Read the model definition and answer for the solid it produces. Units are mm, in the model's axes. A direction names the side the tool comes from. Coordinates: 2 decimals unless noted, no trailing zeros. Write each loop counter-clockwise with the first axis right and the second up, starting at its lowest first coordinate (ties: lowest second). Pieces come first, ordered by that corner, then holes.
(1) Section B-B on z = 63.5 is taken. Write down the section's boundary in (x, y).
(2) Find the intervals of material crossed by probe 1 along Y at (x, z) = (44.5, 27); probe 2 along X at (y, z) = (6, -31); probe 3 along Z at (x, y) = (39, 6), in increasing order.
(3) Which of the six approach directions +Z, -Z, +X, -X, +Y, -Y give full straight-line access (tool end or side, diameter ignored) to faces 1 (the flat face through (25.222, 99.563, -12.21)), 2 (the flat face through (25.49, 77.21, -13.04)), 3 (the flat face through (12.7, 102, -8)), 4 (the flat face through (38.1, 77, -12)), 5 (the flat face through (27.686, 159, 17))?
(4) Given pin 1 (1.6 mm diameter, centred on x = 19, y = 186, fed in from +Z); pin 2 (2 mm diameter, centred on y = 101, z = -7, fed in from +X); pin 3 (5 mm diameter, centred on x = 43.5, z = -43.5, fed in from +Y); pin 4 (1 mm diameter, centred on x = -2, z = -3, fed in from -Y), each flat-ended and moving along its own axis, determine where each tip first touches the part or whether it passes through.
(5) The mould has two halves that part along X. Classify faces 6 (the flat face through (25.22, 74.51, -16.39)), 7 (the cylindrical face through (14.149, 78.337, -20.316)), 8 (the flat face through (19.05, 77, -10)), 9 (the flat face through (31.75, 102, -6)): +X half, -X half, draft (parallel to the pull), parting line (faces both ways), or undercut.
(6) Section A-A on x = 4 is taken. Write down the section's boundary in (y, z) (1 decimal), then the cut area to 3 significant figures.
from build123d import *

# Parameters (mm, degrees)
F1_DEPTH  = 50.8
F2_R      = 31.75
F3_DEPTH  = 50.8
F4_R      = 17.78
F5_R      = 7.62
F6_R      = 1.5875
F7_DEPTH  = 4.7625
F8_W      = 4.572
F8_H      = 86.36
F9_DEPTH  = 127
F11_D     = 3.175
F12_W     = 25.4
F12_H     = 6.35
F13_DEPTH = 15.24
F14_R     = 5.08
F15_W     = 12.7
F15_H     = 6.35
F16_DEPTH = 50.8


with BuildPart() as f1:
    # F0 (on Right) → F1 (new body)
    with BuildSketch(Plane.YZ):
        Polygon((0, 39.7960290042), (0, 0), (-56.4969599977, -124.290533917), (-10.2505199437, -145.3121128855), (50.8, -11.0039709958), (203.2, 14.3960290042), (203.2, 27.0960290042), (50.8, 27.0960290042), (50.8, 39.7960290042), align=None)
    extrude(amount=F1_DEPTH)

    # F2 (on face) → F3 (join)
    with BuildSketch(Plane.XZ):
        with BuildLine():
            Line((0, 45.3162242728), (0, 39.7960290042))
            Line((0, 39.7960290042), (7.3694660021, 39.7960290042))
            ThreePointArc((7.3694660021, 39.7960290042), (25.4, 35.0335290042), (43.4305339979, 39.7960290042))
            Line((43.4305339979, 39.7960290042), (50.8, 39.7960290042))
            Line((50.8, 39.7960290042), (50.8, 45.3162242728))
            ThreePointArc((50.8, 45.3162242728), (25.4, 108.0585290042), (0, 45.3162242728))
        make_face()
        with Locations((25.4, 71.5460290042)):
            Circle(F2_R, mode=Mode.SUBTRACT)
    extrude(amount=-F3_DEPTH)

    # F4
    f4_edges = [f1.edges().sort_by_distance(p)[0] for p in [
        (50.8, -28.24848, -62.145267),
        (0, -28.24848, -62.145267),
        (50.8, 20.27474, -78.158042),
        (0, 20.27474, -78.158042),
    ]]
    fillet(f4_edges, radius=F4_R)

    # F5
    f5_edges = [f1.edges().sort_by_distance(p)[0] for p in [
        (50.8, 127, 1.696029),
        (0, 127, 1.696029),
    ]]
    fillet(f5_edges, radius=F5_R)

    # F6 (on face) → F7 (join)
    with BuildSketch(Plane.XY.offset(27.0960290042)):
        with Locations((19.05, 185.6386214495)):
            Circle(F6_R)
        with Locations((31.75, 185.6386214495)):
            Circle(F6_R)
        with Locations((31.75, 166.5886214495)):
            Circle(F6_R)
        with Locations((19.05, 166.5886214495)):
            Circle(F6_R)
    extrude(amount=F7_DEPTH)

    # F8 (on face) → F9 (cut)
    with BuildSketch(Plane.XY.offset(27.0960290042)):
        with Locations((25.4, 160.02)):
            Rectangle(F8_W, F8_H)
    extrude(amount=-F9_DEPTH, mode=Mode.SUBTRACT)

    # F11 (through all)
    with Locations(Plane.YZ.offset(50.8)):
        with Locations((152.4, 19.4760290042)):
            Hole(F11_D / 2)

    # F12 (on face) → F13 (join)
    with BuildSketch(Plane(origin=(0, 3.157400702, -18.9444042121), x_dir=(1, 0, 0), z_dir=(0, 0.1643989873, -0.9863939238))):
        with Locations((25.4, -99.3757092261)):
            Rectangle(F12_W, F12_H)
        with Locations((25.4, -73.9757092261)):
            Rectangle(F12_W, F12_H)
    extrude(amount=F13_DEPTH)

    # F14
    f14_edges = [f1.edges().sort_by_distance(p)[0] for p in [
        (38.1, 103.686437, -17.639782),
        (38.1, 78.632031, -21.815516),
        (12.7, 78.632031, -21.815516),
        (12.7, 103.686437, -17.639782),
    ]]
    fillet(f14_edges, radius=F14_R)

    # F15 (on face) → F16 (cut)
    with BuildSketch(Plane(origin=(0, 101.1553964653, 16.8592327442), x_dir=(-1, 0, 0), z_dir=(0, 0.9863939238, 0.1643989873))):
        with Locations((-25.4, -22.3807186834)):
            Rectangle(F15_W, F15_H)
    extrude(amount=-F16_DEPTH, mode=Mode.SUBTRACT)


solid = f1.part
Response:
1. outline: (-10.21, 0) - (-5.31, 0) - (-5.31, 50.8) - (-10.21, 50.8) - close; (56.11, 0) - (61.01, 0) - (61.01, 50.8) - (56.11, 50.8) - close
2. probe 1: y = 0 to 203.2
2. probe 2: x = 0 to 50.8
2. probe 3: z = -107.06 to 42.86, 100.24 to 105.43
3. face 1: -Z, +X, -X
3. face 2: none
3. face 3: -Z, -X, +Y
3. face 4: -Z, +X, +Y
3. face 5: +Z, -Z, +Y
4. pin 1: stops at z = 31.86
4. pin 2: stops at x = 38.1
4. pin 3: stops at y = 34.35
4. pin 4: passes through
5. face 6: draft
5. face 7: -X half
5. face 8: undercut
5. face 9: undercut
6. outline: (-50.5, -127) - (-16.2, -142.6) - (43.5, -11.3) - (203.2, 15.3) - (203.2, 27.1) - (50.8, 27.1) - (50.8, 48.1) - (0, 48.1) - (0, -15.8) - close; (0, 95) - (50.8, 95) - (50.8, 101.1) - (0, 101.1) - close; hole circle Ø3.2 at (152.4, 19.5)
6. area: 12,200 mm2
